Could you check a few things on this model? Use its own coordinates, in mm. Face numbers are marked on the shaded views. A direction names the side the tool comes from. Round coordinates to 2 decimals unless told otherwise and drop trailing zeros. Write each loop counter-clockwise with the first axis right and the second up, starting at its lowest first coordinate (ties: lowest second). Pieces come first, ordered by that corner, then holes. Notation, with made-up numbers: (-23, -18.75) - (0, -18.75) arc R17 cw to (0, 14.25) - close; hole circle Ø6 at (28, 28). An arc over 180 degrees is marked (long way). Write each question's results on one line, items separated by ' | '. Start each with the question number.
(1) Imagine slicing it at A-A on z = 11. Write out the boundary of the cut face in (x, y).
(2) For P1, Ø10, axis at x = -37, y = -11.5, coming from the +Z side; P2, Ø10, axis at x = 29, z = 30.5, coming from the -Y side; P3, Ø3, axis at x = 44, y = 8, coming from the +Z side, each with a flat end and sliding along its axis, tell me the tip position at first contact or that it passes through.
(3) Imagine slicing it at D-D on z = 37.5. Write out the boundary of the cut face in (x, y), then the cut area to 3 significant figures.
(4) Please list where these lines run through material, in increasing order: line 1 (Y direction, x = 0, z = 37); line 2 (Y direction, x = 0, z = 24); line 3 (X direction, y = -1.5, z = 39). Write a range as [from, to].
(5) On a 3-axis mill with a long thin cutter (end or side, diameter ignored), from which of +Z, -Z, +X, -X, +Y, -Y can I reach the whole of each face in a straight line? I mean the marked faces 1, 2 and 3. Say none if no direction works.
(6) Thinking about a two-plate mould opening in Y: for the marked faces 4, 5, 6 and 7, which applies, +Y half, -Y half, draft (parallel to the pull), parting line (faces both ways), or undercut?
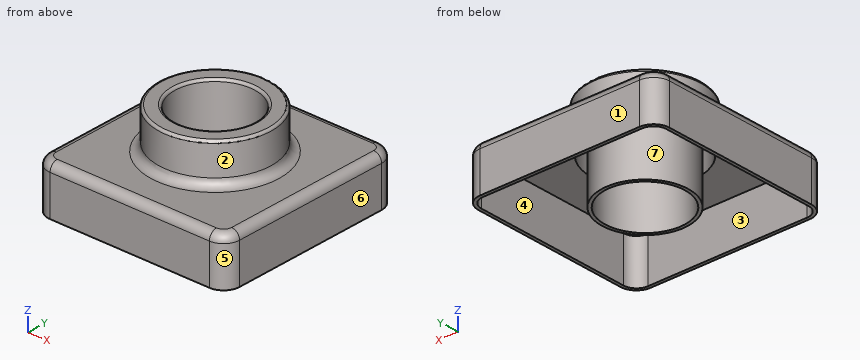
```python
from build123d import *

# Parameters (mm, degrees)
SKETCH3_W           = 120
SKETCH3_H           = 120
BOSS_EXTRUDE1_DEPTH = 30
SKETCH4_R           = 35
BOSS_EXTRUDE2_DEPTH = 25
SKETCH5_R           = 25
CUT_EXTRUDE1_DEPTH  = 102.118742081
FILLET2_R           = 1.5
FILLET3_R           = 10
SHELL1_T            = -2
FILLET4_R           = 5


with BuildPart() as part:
    # Sketch3 → Boss-Extrude1 (new body)
    with BuildSketch(Plane.XY):
        Rectangle(SKETCH3_W, SKETCH3_H)
    extrude(amount=BOSS_EXTRUDE1_DEPTH)

    # Sketch4 → Boss-Extrude2 (add)
    with BuildSketch(Plane.XY.offset(30)):
        Circle(SKETCH4_R)
    extrude(amount=BOSS_EXTRUDE2_DEPTH)

    # Sketch5 → Cut-Extrude1 (cut, through all)
    with BuildSketch(Plane.XY.offset(55)):
        Circle(SKETCH5_R)
    extrude(amount=-CUT_EXTRUDE1_DEPTH, mode=Mode.SUBTRACT)

    # Fillet2
    fillet2_edges = [part.edges().sort_by_distance(p)[0] for p in [
        (-35, 0, 55),
        (-25, 0, 55),
    ]]
    fillet(fillet2_edges, radius=FILLET2_R)

    # Fillet3
    fillet3_edges = [part.edges().sort_by_distance(p)[0] for p in [
        (-60, -60, 15),
        (60, -60, 15),
        (60, 60, 15),
        (-60, 60, 15),
    ]]
    fillet(fillet3_edges, radius=FILLET3_R)

    # Shell1
    shell1_openings = [part.faces().sort_by_distance(p)[0] for p in [
        (0, -58.302943725, 0),
    ]]
    offset(amount=SHELL1_T, openings=shell1_openings, kind=Kind.INTERSECTION)

    # Fillet4
    fillet4_edges = [part.edges().sort_by_distance(p)[0] for p in [
        (-35, 0, 30),
        (-60, 0, 30),
        (0, 60, 30),
        (0, -60, 30),
        (60, 0, 30),
        (57.071067812, 57.071067812, 30),
        (57.071067812, -57.071067812, 30),
        (-57.071067812, -57.071067812, 30),
        (-57.071067812, 57.071067812, 30),
    ]]
    fillet(fillet4_edges, radius=FILLET4_R)


solid = part.part
```
Response:
1) outline: (-60, -50) arc R10 ccw to (-50, -60) - (50, -60) arc R10 ccw to (60, -50) - (60, 50) arc R10 ccw to (50, 60) - (-50, 60) arc R10 ccw to (-60, 50) - close; circle Ø54 at (0, 0); hole (-58, -50) arc R8 ccw to (-50, -58) - (50, -58) arc R8 ccw to (58, -50) - (58, 50) arc R8 ccw to (50, 58) - (-50, 58) arc R8 ccw to (-58, 50) - close; hole circle Ø50 at (0, 0)
2) P1: z = 54.98 | P2: y = -59.97 | P3: z = 30
3) outline: circle Ø70 at (0, 0); circle Ø54 at (0, 0); hole circle Ø66 at (0, 0); hole circle Ø50 at (0, 0) | area: 754 mm²
4) line 1: [-35, -33], [-27, -25], [25, 27], [33, 35] | line 2: [-60, -58], [-27, -25], [25, 27], [58, 60] | line 3: [-34.97, -32.97], [-26.96, -24.95], [24.95, 26.96], [32.97, 34.97]
5) face 1: +Z, -Z, +X, -X, +Y | face 2: +Z | face 3: -Z
6) face 4: undercut | face 5: -Y half | face 6: draft | face 7: undercut
